from build123d import *

# Parameters (mm, degrees)
SKETCH1_W           = 240
SKETCH1_H           = 151
BOSS_EXTRUDE1_DEPTH = 5
SKETCH3_W           = 13
SKETCH3_H           = 57
CUT_EXTRUDE2_DEPTH  = 10
SKETCH5_W           = 5.2
SKETCH5_H           = 20.2
CUT_EXTRUDE4_DEPTH  = 10
SKETCH6_R           = 2
CUT_EXTRUDE5_DEPTH  = 10
SKETCH7_R           = 2
CUT_EXTRUDE6_DEPTH  = 10
CUT_EXTRUDE7_DEPTH  = 10
SKETCH9_R           = 2
CUT_EXTRUDE8_DEPTH  = 10
SKETCH10_R          = 4
SKETCH10_R_2        = 2
BOSS_EXTRUDE2_DEPTH = 5
CUT_EXTRUDE10_DEPTH = 10
SKETCH13_W          = 30
SKETCH13_H          = 35
CUT_EXTRUDE11_DEPTH = 10
SKETCH16_R          = 2
CUT_EXTRUDE13_DEPTH = 5
CUT_EXTRUDE14_DEPTH = 5
CUT_EXTRUDE15_DEPTH = 5
SKETCH20_W          = 5.2
SKETCH20_H          = 20.2
CUT_EXTRUDE17_DEPTH = 10
SKETCH21_R          = 2
CUT_EXTRUDE18_DEPTH = 10
CUT_EXTRUDE20_DEPTH = 5
SKETCH25_R          = 2
CUT_EXTRUDE21_DEPTH = 5
SKETCH26_R          = 2
CUT_EXTRUDE22_DEPTH = 10
SKETCH27_R          = 4
SKETCH27_R_2        = 2
BOSS_EXTRUDE4_DEPTH = 5
FILLET1_R           = 14
SKETCH28_W          = 5.2
SKETCH28_H          = 20.2
CUT_EXTRUDE23_DEPTH = 5
SKETCH29_W          = 20.2
SKETCH29_H          = 5.2
CUT_EXTRUDE24_DEPTH = 5
SKETCH30_R          = 2
CUT_EXTRUDE25_DEPTH = 5
SKETCH31_R          = 4
SKETCH31_R_2        = 2
BOSS_EXTRUDE5_DEPTH = 5
SKETCH32_R          = 2
CUT_EXTRUDE26_DEPTH = 5
SKETCH33_W          = 5
SKETCH33_H          = 30
SKETCH33_H_2        = 20
BOSS_EXTRUDE6_DEPTH = 5
SKETCH34_R          = 2.25
CUT_EXTRUDE27_DEPTH = 5
CUT_EXTRUDE28_DEPTH = 5
SKETCH36_R          = 2
CUT_EXTRUDE29_DEPTH = 5


with BuildPart() as part:
    # Sketch1 → Boss-Extrude1 (new body)
    with BuildSketch(Plane.XY):
        Rectangle(SKETCH1_W, SKETCH1_H)
    extrude(amount=BOSS_EXTRUDE1_DEPTH)

    # Sketch3 → Cut-Extrude2 (cut)
    with BuildSketch(Plane(origin=(0, 0, 0), x_dir=(-1, 0, 0), z_dir=(0, 0, -1))):
        with Locations((0, -47)):
            Rectangle(SKETCH3_W, SKETCH3_H)
    extrude(amount=-CUT_EXTRUDE2_DEPTH, mode=Mode.SUBTRACT)

    # Sketch5 → Cut-Extrude4 (cut)
    with BuildSketch(Plane(origin=(0, 0, 0), x_dir=(-1, 0, 0), z_dir=(0, 0, -1))):
        with Locations((-34.4, -53.2)):
            Rectangle(SKETCH5_W, SKETCH5_H)
        with Locations((34.4, -53.2)):
            Rectangle(SKETCH5_W, SKETCH5_H)
    extrude(amount=-CUT_EXTRUDE4_DEPTH, mode=Mode.SUBTRACT)

    # Sketch6 → Cut-Extrude5 (cut)
    with BuildSketch(Plane(origin=(0, 0, 0), x_dir=(-1, 0, 0), z_dir=(0, 0, -1))):
        with Locations((11.5, 19.5)):
            Circle(SKETCH6_R)
        with Locations((11.5, 1.5)):
            Circle(SKETCH6_R)
        with Locations((11.5, -16.5)):
            Circle(SKETCH6_R)
        with Locations((-11.5, -16.5)):
            Circle(SKETCH6_R)
        with Locations((-11.5, 1.5)):
            Circle(SKETCH6_R)
        with Locations((-11.5, 19.5)):
            Circle(SKETCH6_R)
    extrude(amount=-CUT_EXTRUDE5_DEPTH, mode=Mode.SUBTRACT)

    # Sketch7 → Cut-Extrude6 (cut)
    with BuildSketch(Plane(origin=(0, 0, 0), x_dir=(-1, 0, 0), z_dir=(0, 0, -1))):
        with Locations((-43, -2.1)):
            Circle(SKETCH7_R)
        with Locations((-43, -17.6)):
            Circle(SKETCH7_R)
        with Locations((-29, -17.6)):
            Circle(SKETCH7_R)
        with Locations((-29, -2.1)):
            Circle(SKETCH7_R)
    extrude(amount=-CUT_EXTRUDE6_DEPTH, mode=Mode.SUBTRACT)

    # Sketch8 → Cut-Extrude7 (cut)
    with BuildSketch(Plane(origin=(0, 0, 0), x_dir=(-1, 0, 0), z_dir=(0, 0, -1))):
        with BuildLine():
            Line((-120, -26.5), (-92, -26.5))
            ThreePointArc((-92, -26.5), (-72, -46.5), (-92, -66.5))
            Line((-92, -66.5), (-120, -66.5))
            Line((-120, -66.5), (-120, -26.5))
        make_face()
    extrude(amount=-CUT_EXTRUDE7_DEPTH, mode=Mode.SUBTRACT)

    # Sketch9 → Cut-Extrude8 (cut)
    with BuildSketch(Plane(origin=(0, 0, 0), x_dir=(-1, 0, 0), z_dir=(0, 0, -1))):
        with Locations((-59.2, -21.5)):
            Circle(SKETCH9_R)
        with Locations((-107.8, -21.5)):
            Circle(SKETCH9_R)
        with Locations((-49.2, -73)):
            Circle(SKETCH9_R)
        with Locations((-107.8, -73)):
            Circle(SKETCH9_R)
    extrude(amount=-CUT_EXTRUDE8_DEPTH, mode=Mode.SUBTRACT)

    # Sketch10 → Boss-Extrude2 (add)
    with BuildSketch(Plane(origin=(0, 0, 0), x_dir=(-1, 0, 0), z_dir=(0, 0, -1))):
        with Locations((-107.8, -73)):
            Circle(SKETCH10_R)
        with Locations((-107.8, -73)):
            Circle(SKETCH10_R_2, mode=Mode.SUBTRACT)
        with Locations((-49.2, -73)):
            Circle(SKETCH10_R)
        with Locations((-49.2, -73)):
            Circle(SKETCH10_R_2, mode=Mode.SUBTRACT)
    extrude(amount=-BOSS_EXTRUDE2_DEPTH)

    # Sketch12 → Cut-Extrude10 (cut)
    with BuildSketch(Plane(origin=(0, 0, 0), x_dir=(-1, 0, 0), z_dir=(0, 0, -1))):
        with BuildLine():
            Line((-45.2, -35.107061825), (-45.2, -60.107061825))
            ThreePointArc((-45.2, -60.107061825), (-49.2, -64.107061825), (-53.2, -60.107061825))
            Line((-53.2, -60.107061825), (-53.2, -35.107061825))
            ThreePointArc((-53.2, -35.107061825), (-49.2, -31.107061825), (-45.2, -35.107061825))
        make_face()
    extrude(amount=-CUT_EXTRUDE10_DEPTH, mode=Mode.SUBTRACT)

    # Sketch13 → Cut-Extrude11 (cut)
    with BuildSketch(Plane(origin=(0, 0, 0), x_dir=(-1, 0, 0), z_dir=(0, 0, -1))):
        with Locations((-105, 58)):
            Rectangle(SKETCH13_W, SKETCH13_H)
        with Locations((105, 58)):
            Rectangle(SKETCH13_W, SKETCH13_H)
    extrude(amount=-CUT_EXTRUDE11_DEPTH, mode=Mode.SUBTRACT)

    # Sketch16 → Cut-Extrude13 (cut)
    with BuildSketch(Plane(origin=(0, 0, 0), x_dir=(-1, 0, 0), z_dir=(0, 0, -1))):
        with Locations((59, -29.5)):
            Circle(SKETCH16_R)
        with Locations((59, -60.5)):
            Circle(SKETCH16_R)
    extrude(amount=-CUT_EXTRUDE13_DEPTH, mode=Mode.SUBTRACT)

    # Sketch17 → Cut-Extrude14 (cut)
    with BuildSketch(Plane(origin=(0, 0, 0), x_dir=(-1, 0, 0), z_dir=(0, 0, -1))):
        with BuildLine():
            Line((-95, 17), (-95, -3))
            ThreePointArc((-95, -3), (-100, -8), (-105, -3))
            Line((-105, -3), (-105, 17))
            ThreePointArc((-105, 17), (-100, 22), (-95, 17))
        make_face()
    extrude(amount=-CUT_EXTRUDE14_DEPTH, mode=Mode.SUBTRACT)

    # Sketch18 → Cut-Extrude15 (cut)
    with BuildSketch(Plane(origin=(0, 0, 0), x_dir=(-1, 0, 0), z_dir=(0, 0, -1))):
        with BuildLine():
            Line((67, -15.5), (67, 4.5))
            ThreePointArc((67, 4.5), (72, 9.5), (77, 4.5))
            Line((77, 4.5), (77, -15.5))
            ThreePointArc((77, -15.5), (72, -20.5), (67, -15.5))
        make_face()
    extrude(amount=-CUT_EXTRUDE15_DEPTH, mode=Mode.SUBTRACT)

    # Sketch20 → Cut-Extrude17 (cut)
    with BuildSketch(Plane(origin=(0, 0, 0), x_dir=(-1, 0, 0), z_dir=(0, 0, -1))):
        with Locations((58.395562695, 28.1)):
            Rectangle(SKETCH20_W, SKETCH20_H)
    extrude(amount=-CUT_EXTRUDE17_DEPTH, mode=Mode.SUBTRACT)

    # Sketch21 → Cut-Extrude18 (cut)
    with BuildSketch(Plane(origin=(0, 0, 0), x_dir=(-1, 0, 0), z_dir=(0, 0, -1))):
        with Locations((58.295562695, -7.3)):
            Circle(SKETCH21_R)
        with Locations((58.295562695, 63.3)):
            Circle(SKETCH21_R)
    extrude(amount=-CUT_EXTRUDE18_DEPTH, mode=Mode.SUBTRACT)

    # Sketch24 → Cut-Extrude20 (cut)
    with BuildSketch(Plane.XY.offset(5)):
        Polygon((66.2, -45.5), (66.196152437, -25.300000366), (61, -25.5), (61, -45.5), align=None)
    extrude(amount=-CUT_EXTRUDE20_DEPTH, mode=Mode.SUBTRACT)

    # Sketch25 → Cut-Extrude21 (cut)
    with BuildSketch(Plane(origin=(0, 0, 0), x_dir=(-1, 0, 0), z_dir=(0, 0, -1))):
        with Locations((-63.5, -68.3)):
            Circle(SKETCH25_R)
    extrude(amount=-CUT_EXTRUDE21_DEPTH, mode=Mode.SUBTRACT)

    # Sketch26 → Cut-Extrude22 (cut)
    with BuildSketch(Plane(origin=(0, 0, 0), x_dir=(-1, 0, 0), z_dir=(0, 0, -1))):
        with Locations((39.8, 73)):
            Circle(SKETCH26_R)
        with Locations((-12.2, 73)):
            Circle(SKETCH26_R)
    extrude(amount=-CUT_EXTRUDE22_DEPTH, mode=Mode.SUBTRACT)

    # Sketch27 → Boss-Extrude4 (add)
    with BuildSketch(Plane(origin=(0, 0, 0), x_dir=(-1, 0, 0), z_dir=(0, 0, -1))):
        with Locations((39.8, 73)):
            Circle(SKETCH27_R)
        with Locations((39.8, 73)):
            Circle(SKETCH27_R_2, mode=Mode.SUBTRACT)
        with Locations((-12.2, 73)):
            Circle(SKETCH27_R)
        with Locations((-12.2, 73)):
            Circle(SKETCH27_R_2, mode=Mode.SUBTRACT)
    extrude(amount=-BOSS_EXTRUDE4_DEPTH)

    # Fillet1
    fillet1_edges = [part.edges().sort_by_distance(p)[0] for p in [
        (120, 40.5, 2.5),
        (-120, 40.5, 2.5),
    ]]
    fillet(fillet1_edges, radius=FILLET1_R)

    # Sketch28 → Cut-Extrude23 (cut)
    with BuildSketch(Plane.XY.offset(5)):
        with Locations((22.4, 43.1)):
            Rectangle(SKETCH28_W, SKETCH28_H)
    extrude(amount=-CUT_EXTRUDE23_DEPTH, mode=Mode.SUBTRACT)

    # Sketch29 → Cut-Extrude24 (cut)
    with BuildSketch(Plane.XY.offset(5)):
        with Locations((57.4, 13.3)):
            Rectangle(SKETCH29_W, SKETCH29_H)
    extrude(amount=-CUT_EXTRUDE24_DEPTH, mode=Mode.SUBTRACT)

    # Sketch30 → Cut-Extrude25 (cut)
    with BuildSketch(Plane(origin=(0, 0, 0), x_dir=(-1, 0, 0), z_dir=(0, 0, -1))):
        with Locations((-79.8, 73)):
            Circle(SKETCH30_R)
    extrude(amount=-CUT_EXTRUDE25_DEPTH, mode=Mode.SUBTRACT)

    # Sketch31 → Boss-Extrude5 (add)
    with BuildSketch(Plane(origin=(0, 0, 0), x_dir=(-1, 0, 0), z_dir=(0, 0, -1))):
        with Locations((-79.8, 73)):
            Circle(SKETCH31_R)
        with Locations((-79.8, 73)):
            Circle(SKETCH31_R_2, mode=Mode.SUBTRACT)
    extrude(amount=-BOSS_EXTRUDE5_DEPTH)

    # Sketch32 → Cut-Extrude26 (cut)
    with BuildSketch(Plane(origin=(0, 0, 0), x_dir=(-1, 0, 0), z_dir=(0, 0, -1))):
        with Locations((82.999989356, 38)):
            Circle(SKETCH32_R)
    extrude(amount=-CUT_EXTRUDE26_DEPTH, mode=Mode.SUBTRACT)

    # Sketch33 → Boss-Extrude6 (add)
    with BuildSketch(Plane(origin=(0, 0, 0), x_dir=(-1, 0, 0), z_dir=(0, 0, -1))):
        with Locations((122.5, -4.5)):
            Rectangle(SKETCH33_W, SKETCH33_H)
        with Locations((-122.5, -6.5)):
            Rectangle(SKETCH33_W, SKETCH33_H_2)
    extrude(amount=-BOSS_EXTRUDE6_DEPTH)

    # Sketch34 → Cut-Extrude27 (cut)
    with BuildSketch(Plane(origin=(0, 0, 0), x_dir=(-1, 0, 0), z_dir=(0, 0, -1))):
        with Locations((113.98, -48)):
            Circle(SKETCH34_R)
        with Locations((69.98, -48)):
            Circle(SKETCH34_R)
    extrude(amount=-CUT_EXTRUDE27_DEPTH, mode=Mode.SUBTRACT)

    # Sketch35 → Cut-Extrude28 (cut)
    with BuildSketch(Plane(origin=(0, 0, 0), x_dir=(-1, 0, 0), z_dir=(0, 0, -1))):
        Polygon((-120, 14.605611853), (-117, 14.605611853), (-117, 16.105611853), (-113.7, 16.105611853), (-113.7, 14.605611853), (-109.705118332, 14.605611853), (-109.705118332, 10.205611853), (-113.7, 10.205611853), (-113.7, 8.705611853), (-117, 8.705611853), (-117, 10.205611853), (-120, 10.205611853), align=None)
        Polygon((100, -24.37851787), (111.7, -24.37851787), (111.7, -22.87851787), (115, -22.87851787), (115, -24.37851787), (120, -24.37851787), (120, -28.77851787), (115, -28.77851787), (115, -30.27851787), (111.7, -30.27851787), (111.7, -28.77851787), (100, -28.77851787), align=None)
    extrude(amount=-CUT_EXTRUDE28_DEPTH, mode=Mode.SUBTRACT)

    # Sketch36 → Cut-Extrude29 (cut)
    with BuildSketch(Plane(origin=(0, 0, 0), x_dir=(-1, 0, 0), z_dir=(0, 0, -1))):
        with Locations((-22.5, 65.3)):
            Circle(SKETCH36_R)
    extrude(amount=-CUT_EXTRUDE29_DEPTH, mode=Mode.SUBTRACT)


solid = part.part
Here's how the part is built. I have some questions about the finished solid (model axes, mm). A direction names the side the tool comes from. Give positions to 0.01 mm unless a question says otherwise; leave off trailing zeros. Order: outer loops, then holes, each group sorted by start corner. A loop starts at its lowest first (then second) coordinate and runs counter-clockwise, first axis right, second up. Notation, with made-up numbers: M -31,-20 L -27,-20 A36 cw -27,16 Z; hole C 89.5,82 d2. An arc over 180 degrees is marked long. Answer as a JSON object with one key per item and string values. Group by question number.
1) Please list where these lines run through material, in increasing order: L1, parallel to Y at x = 43, z = 2.45; L2, parallel to Y at x = 59.2, z = 1.8; L3, parallel to X at y = -6.5, z = 2.9. Write a range as [from, to].
2) I'm going to push flat-ended pins straight in: pin 1 Ø3.5 at (x, y) = (-11.5, 1.5) entering from +Z; pin 2 Ø0.9 at (x, z) = (118.5, 3) entering from +Y; pin 3 Ø1.5 at (y, z) = (13.5, 2) entering from -X; pin 4 Ø2.5 at (y, z) = (59, 3.5) entering from +X. Where does each tip first touch, or does it pass through?
3) We'd pull the mould along X, two halves only. Please class faces 1 (the flat face through (120, 7, 2)), 2 (the cylindrical face through (107.9, -77, 2.5)), 3 (the flat face through (115, -75.5, 2)), 4 (the flat face through (-34, -43.1, 2)): pulls with the +X half, pulls with the -X half, needs draft (parallel to the pull), parting line crosses it, or undercut.
4) On a 3-axis mill with a long thin cutter (end or side, diameter ignored), from which of +Z, -Z, +X, -X, +Y, -Y can I reach the whole of each face in a straight line? I mean faces 5 (the flat face through (86, 75.5, 2)), 6 (the flat face through (120, -22, 2)), 7 (the flat face through (-118, -28.779, 2)), 8 (the flat face through (-31.8, -53, 2)). Say none if no direction works.
5) Suppose I cut it at C-C, the plane x = -26. Write out the boundary of the cut face in (y, z), plus the area to 3 significant figures.
6) Suppose I cut it at B-B, the plane z = 1.15. Count the separate pieces of the cut face and the enclosed holes in it, plus the area to 3 significant figures.
7) Suppose I cut it at A-A, the plane y = 45.5. Write out the boundary of the cut face in (x, z), plus the area to 3 significant figures.
Results found:
{
 "1": {"L1": "[-75.5, -19.6], [-15.6, -4.1], [-0.1, 75.5]", "L2": "[-75.5, -23.5], [-19.5, 10.7], [15.9, 75.5]", "L3": "[-125, -77], [-67, -60.13], [-56.46, 96.43], [103.57, 125]"},
 "2": {"pin 1": "through", "pin 2": "y = 33.63", "pin 3": "x = -120", "pin 4": "x = 90"},
 "3": {"face 1": "pulls with the +X half", "face 2": "undercut", "face 3": "needs draft", "face 4": "undercut"},
 "4": {"face 5": "+Z, -Z, +X, +Y", "face 6": "+Z, -Z, +X, -Y", "face 7": "+Z, -Z, -X", "face 8": "+Z, -Z"},
 "5": {"outline": "M -75.5,0 L 75.5,0 L 75.5,5 L -75.5,5 Z", "area": "755 mm²"},
 "6": {"separate pieces": "1", "enclosed holes": "35", "area": "29,900 mm²"},
 "7": {"outline": "M -90,0 L 19.8,0 L 19.8,5 L -90,5 Z; M 25,0 L 90,0 L 90,5 L 25,5 Z", "area": "874 mm²"}
}
